Geometry check sheet. Reference: the model listing, model coordinates, mm. A direction names the side the tool comes from. Coordinates: 2 decimals unless noted, no trailing zeros. Order: outer loops, then holes, each group sorted by start corner. A loop starts at its lowest first (then second) coordinate and runs counter-clockwise, first axis right, second up.
```python
from build123d import *

# Parameters (mm, degrees)
F1_DEPTH = 209.55
F2_W     = 20.6375
F2_H     = 20.6375
F2_W_2   = 20.6374746
F2_W_3   = 69.85
F2_H_2   = 55.5625
F2_W_4   = 26.19375
F2_H_3   = 26.19375
F3_DEPTH = 0.4064


# Not quite as in the source:
# - the dataset's text gives a spline's control points without its knots; the knots are read off the source's solid


with BuildPart() as f1:
    # F0 (on Right) → F1 (new body, symmetric)
    with BuildSketch(Plane.YZ):
        Polygon((-139.7, 0), (0, 0), (0, 50.8), (-139.2936, 50.8), (-139.2936, 51.054), (-40.6298144724, 149.7177855276), (-40.9171826682, 150.0051537235), (-139.7, 51.2223363917), align=None)
    extrude(amount=F1_DEPTH, both=True)

    # F2 (on face) → F3 (cut, through all)
    with BuildSketch(Plane(origin=(0, -95.4611681959, 95.4611681959), x_dir=(1, 0, 0), z_dir=(0, -0.7071067812, 0.7071067812))):
        with Locations((-43.1144662619, 12.8675024964)):
            Rectangle(F2_W, F2_H)
        with Locations((-43.5109856619, 41.4425024964)):
            Rectangle(F2_W, F2_H)
        with Locations((-9.7769662619, 12.8675024964)):
            Rectangle(F2_W, F2_H)
        with Locations((-10.1734983619, 41.4425024964)):
            Rectangle(F2_W_2, F2_H)
        with Locations((158.1011587381, 30.3300024964)):
            Rectangle(F2_W_3, F2_H_2)
        with Locations((94.6011587381, 15.6456274964)):
            Rectangle(F2_W_4, F2_H_3)
        with BuildLine():
            add(Edge.make_bspline(
                [(21.8352387381, 39.0695074964), (20.5863715381, 40.3187048964), (18.8311045381, 41.0456274964), (17.0644329381, 41.0456274964)],
                knots=[7, 7, 7, 7, 8, 8, 8, 8], degree=3))
            add(Edge.make_bspline(
                [(17.0644329381, 41.0456274964), (15.2984979381, 41.0456274964), (13.5432309381, 40.3187048964), (12.2940335381, 39.0695074964)],
                knots=[0, 0, 0, 0, 1, 1, 1, 1], degree=3))
            add(Edge.make_bspline(
                [(12.2940335381, 39.0695074964), (11.0451663381, 37.8209958964), (10.3175579381, 36.0653986964), (10.3175579381, 34.2987524964), (10.3175579381, 32.5327920964), (11.0451663381, 30.7771440964), (12.2940335381, 29.5279720964)],
                knots=[1, 1, 1, 1, 2, 2, 2, 3, 3, 3, 3], degree=3))
            add(Edge.make_bspline(
                [(12.2940335381, 29.5279720964), (13.5432309381, 28.2794858964), (15.2984979381, 27.5518774964), (17.0644329381, 27.5518774964), (18.8311045381, 27.5518774964), (20.5863715381, 28.2794858964), (21.8352387381, 29.5279720964)],
                knots=[3, 3, 3, 3, 4, 4, 4, 5, 5, 5, 5], degree=3))
            add(Edge.make_bspline(
                [(21.8352387381, 29.5279720964), (23.0844107381, 30.7771440964), (23.8113079381, 32.5327920964), (23.8113079381, 34.2987524964), (23.8113079381, 36.0653986964), (23.0844107381, 37.8209958964), (21.8352387381, 39.0695074964)],
                knots=[5, 5, 5, 5, 6, 6, 6, 7, 7, 7, 7], degree=3))
        make_face()
        with BuildLine():
            add(Edge.make_bspline(
                [(-87.3753632619, 38.4569864964), (-91.2690054619, 42.3506286964), (-96.7418418619, 44.6175024964), (-102.2488412619, 44.6175024964)],
                knots=[7, 7, 7, 7, 8, 8, 8, 8], degree=3))
            add(Edge.make_bspline(
                [(-102.2488412619, 44.6175024964), (-107.7551548619, 44.6175024964), (-113.2283468619, 42.3506286964), (-117.1219890619, 38.4569864964)],
                knots=[0, 0, 0, 0, 1, 1, 1, 1], degree=3))
            add(Edge.make_bspline(
                [(-117.1219890619, 38.4569864964), (-121.0156820619, 34.5633442964), (-123.2832162619, 29.0904570964), (-123.2832162619, 23.5831274964), (-123.2832162619, 18.0764836964), (-121.0156820619, 12.6035964964), (-117.1219890619, 8.7092430964)],
                knots=[1, 1, 1, 1, 2, 2, 2, 3, 3, 3, 3], degree=3))
            add(Edge.make_bspline(
                [(-117.1219890619, 8.7092430964), (-113.2283468619, 4.8156008964), (-107.7551548619, 2.5487524964), (-102.2488412619, 2.5487524964), (-96.7418418619, 2.5487524964), (-91.2690054619, 4.8156008964), (-87.3753632619, 8.7092430964)],
                knots=[3, 3, 3, 3, 4, 4, 4, 5, 5, 5, 5], degree=3))
            add(Edge.make_bspline(
                [(-87.3753632619, 8.7092430964), (-83.4813654619, 12.6035964964), (-81.2144662619, 18.0764836964), (-81.2144662619, 23.5831274964), (-81.2144662619, 29.0904570964), (-83.4813654619, 34.5633442964), (-87.3753632619, 38.4569864964)],
                knots=[5, 5, 5, 5, 6, 6, 6, 7, 7, 7, 7], degree=3))
        make_face()
        with BuildLine():
            add(Edge.make_bspline(
                [(-157.2253632619, 38.4569864964), (-161.1190054619, 42.3506286964), (-166.5918418619, 44.6175024964), (-172.0988412619, 44.6175024964)],
                knots=[7, 7, 7, 7, 8, 8, 8, 8], degree=3))
            add(Edge.make_bspline(
                [(-172.0988412619, 44.6175024964), (-177.6051548619, 44.6175024964), (-183.0781690619, 42.3506286964), (-186.9721668619, 38.4569864964), (-190.8661646619, 34.5633442964), (-193.1332162619, 29.0904570964), (-193.1332162619, 23.5831274964), (-193.1332162619, 18.0764836964), (-190.8661646619, 12.6035964964), (-186.9721668619, 8.7092430964)],
                knots=[0, 0, 0, 0, 1, 1, 1, 2, 2, 2, 3, 3, 3, 3], degree=3))
            add(Edge.make_bspline(
                [(-186.9721668619, 8.7092430964), (-183.0781690619, 4.8156008964), (-177.6051548619, 2.5487524964), (-172.0988412619, 2.5487524964), (-166.5918418619, 2.5487524964), (-161.1190054619, 4.8156008964), (-157.2253632619, 8.7092430964)],
                knots=[3, 3, 3, 3, 4, 4, 4, 5, 5, 5, 5], degree=3))
            add(Edge.make_bspline(
                [(-157.2253632619, 8.7092430964), (-153.3313654619, 12.6035964964), (-151.0644662619, 18.0764836964), (-151.0644662619, 23.5831274964), (-151.0644662619, 29.0904570964), (-153.3313654619, 34.5633442964), (-157.2253632619, 38.4569864964)],
                knots=[5, 5, 5, 5, 6, 6, 6, 7, 7, 7, 7], degree=3))
        make_face()
        with BuildLine():
            add(Edge.make_bspline(
                [(69.5828445381, 40.1919080964), (68.0401501381, 41.7353136964), (65.8721585381, 42.6331274964), (63.6896889381, 42.6331274964)],
                knots=[7, 7, 7, 7, 8, 8, 8, 8], degree=3))
            add(Edge.make_bspline(
                [(63.6896889381, 42.6331274964), (61.5075495381, 42.6331274964), (59.3392023381, 41.7353136964), (57.7965079381, 40.1919080964)],
                knots=[0, 0, 0, 0, 1, 1, 1, 1], degree=3))
            add(Edge.make_bspline(
                [(57.7965079381, 40.1919080964), (56.2534579381, 38.6492136964), (55.3553139381, 36.4808664964), (55.3553139381, 34.2987524964), (55.3553139381, 32.1166130964), (56.2534579381, 29.9482658964), (57.7965079381, 28.4055714964)],
                knots=[1, 1, 1, 1, 2, 2, 2, 3, 3, 3, 3], degree=3))
            add(Edge.make_bspline(
                [(57.7965079381, 28.4055714964), (59.3392023381, 26.8628262964), (61.5075495381, 25.9643774964), (63.6896889381, 25.9643774964), (65.8721585381, 25.9643774964), (68.0401501381, 26.8628262964), (69.5828445381, 28.4055714964)],
                knots=[3, 3, 3, 3, 4, 4, 4, 5, 5, 5, 5], degree=3))
            add(Edge.make_bspline(
                [(69.5828445381, 28.4055714964), (71.1259453381, 29.9482658964), (72.0240639381, 32.1166130964), (72.0240639381, 34.2987524964), (72.0240639381, 36.4808664964), (71.1259453381, 38.6492136964), (69.5828445381, 40.1919080964)],
                knots=[5, 5, 5, 5, 6, 6, 6, 7, 7, 7, 7], degree=3))
        make_face()
    extrude(amount=-F3_DEPTH, mode=Mode.SUBTRACT)


solid = f1.part
```
Item 1: Sectioned sample at C-C (y = -128). Record the cut outline in (x, z).
Item 2: Sectioned sample at B-B (x = 137.5). Record the cut outline in (y, z).
Item 3: Thickness scan on line 1 along Z through (x, y) = (-171.5, -70.5); line 2 along Z through (x, y) = (-103.5, -103.5); line 3 along Z through (x, y) = (179, -119.5). Record the ranges inside material, lowest first.
Item 4: Sectioned sample at D-D (x = -135). Record the cut outline in (y, z), and give its area (3 significant figures).
Item 5: Sectioned sample at A-A (x = -7). Record the cut outline in (y, z), and give its area (3 significant figures).
Item 6: Release check for a two-part mould opening along X. For faces 4 (the face through (3, -69, 50.8)), 5 (the face through (81.504, -84.4, 106.3)), 6 (the face through (209.55, -70, 31)), 7 (the face through (-209.55, -70, 31)) record: pulls with the +X half, pulls with the -X half, needs draft (parallel to the pull), parting line crosses it, or undercut.
Item 7: Depth check by flat-ended pin: P1, Ø2, axis at x = 57.5, y = -93, coming from the +Z side; P2, Ø4.5, axis at y = -84, z = 101.5, coming from the -X side; P3, Ø6, axis at x = -161, y = -51, coming from the +Z side; P4, Ø8, axis at x = -144, z = 117, coming from the -Y side. Enter the tip coordinate at first touch or a pass-through.
Item 8: Tool access check on faces 1 (the face through (123.176, -74.1, 116.5)), 2 (the face through (3, 0, 25)), 3 (the face through (2.93, -90.65, 99.7)). Record the directions out of +Z, -Z, +X, -X, +Y, -Y that give a thin tool (end or side, any length) a straight path to the whole face; none if there is none.
Geometry check:
1. outline: (-209.55, 0) - (209.55, 0) - (209.55, 50.8) - (-209.55, 50.8) - close; (-209.55, 62.35) - (209.55, 62.35) - (209.55, 62.92) - (-209.55, 62.92) - close
2. outline: (-139.7, 0) - (0, 0) - (0, 50.8) - (-139.29, 50.8) - (-139.29, 51.05) - (-93.37, 96.98) - (-93.66, 97.26) - (-139.7, 51.22) - close; (-54.37, 136.55) - (-54.08, 136.26) - (-40.63, 149.72) - (-40.92, 150.01) - close
3. line 1: z = 0 to 50.8
3. line 2: z = 0 to 50.8, 86.85 to 87.42
3. line 3: z = 0 to 50.8, 70.85 to 71.42
4. outline: (-139.7, 0) - (0, 0) - (0, 50.8) - (-139.29, 50.8) - (-139.29, 51.05) - (-40.63, 149.72) - (-40.92, 150.01) - (-139.7, 51.22) - close
4. area: 7,150 mm2
5. outline: (-139.7, 0) - (0, 0) - (0, 50.8) - (-139.29, 50.8) - (-139.29, 51.05) - (-93.37, 96.98) - (-93.66, 97.26) - (-139.7, 51.22) - close; (-79.07, 111.86) - (-78.78, 111.57) - (-73.17, 117.18) - (-73.45, 117.47) - close; (-58.86, 132.06) - (-58.57, 131.77) - (-40.63, 149.72) - (-40.92, 150.01) - close
5. area: 7,140 mm2
6. face 4: needs draft
6. face 5: undercut
6. face 6: pulls with the +X half
6. face 7: pulls with the -X half
7. P1: stops at z = 98.92
7. P2: passes through
7. P3: stops at z = 142.92
7. P4: stops at y = -77.92
8. face 1: +Z, +Y, -Y
8. face 2: +Z, -Z, +X, -X, +Y
8. face 3: +X, -X, +Y
